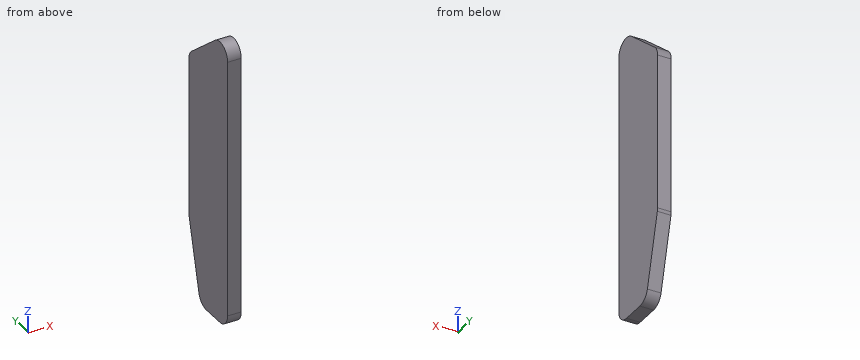
Autodesk Inventor part; units mm, degrees
ref_plane "YZ Plane" through (0, 0, 0) normal (1, 0, 0) x (0, 1, 0)
ref_plane "XZ Plane" through (0, 0, 0) normal (0, 1, 0) x (-1, 0, 0)
ref_plane "XY Plane" through (0, 0, 0) normal (0, 0, 1) x (1, 0, 0)
sketch "Sketch1" plane through (0, 0, 0) normal (1, 0, 0) x (0, 1, 0)
  line L0 (-15.875, 69.85) -> (15.875, 69.85)
  line L1 (15.875, 69.85) -> (15.875, -69.85)
  line L2 (15.875, -69.85) -> (-15.875, -69.85)
  line L3 (-15.875, -69.85) -> (-15.875, 69.85)
  line L4 (-15.875, 69.85) -> (15.875, -69.85) construction
  line L5 (15.875, 69.85) -> (-15.875, -69.85) construction
  line L6 (-15.875, 69.85) -> (15.875, 44.45)
  point P0 (0, 0)
  dimension "d0" = 31.75
  dimension "d1" = 139.7
  dimension "d2" = 25.4
extrude "Extrusion1" add sketch "Sketch1" along normal blind 6.35 contours L6 L1 L2 L3
chamfer "Chamfer1" distance 9.525 distance2 38.1 1 edges at (3.175, 15.875, -69.85) measured on face at (4.2333, -5.2917, -69.85)
fillet "Fillet1" radius 6.35 4 edges at (3.175, -15.875, 69.85) (3.175, 15.875, -31.75) (3.175, 6.35, -69.85) (3.175, -15.875, -69.85)
fillet "Fillet2" radius 6.35 1 edges at (3.175, 15.875, 44.45)
properties part number "Wheel Guards" material "UHMW, White"
Check sheet for the modelled part. Datum: model origin and axes. Units: mm. Coordinates: 2 decimals unless noted, no trailing zeros. Write each loop counter-clockwise with the first axis right and the second up, starting at its lowest first coordinate (ties: lowest second). Pieces come first, ordered by that corner, then holes. Notation, with made-up numbers: (-2, -25) - (5, -25) arc R25 cw to (5, -8) - close; hole circle Ø11 at (49.25, -12.75). An arc over 180 degrees is marked (long way). One line per question, with ' | ' between items.
Item 1: Gauge pin test, flat end, axial feed: P1, Ø1.5, axis at x = 3.5, z = -44.5, coming from the +Y side (3 decimals). Record the tip position at first contact, or that the pin passes through.
Determined:
P1: stops at y = 12.875
Item 2: Sectioned sample at A-A on x = 2. Record the boundary of the cut face in (y, z) (3 decimals), plus the area to 3 significant figures.
Determined:
outline: (-15.875, -63.5) arc R6.35 ccw to (-9.525, -69.85) - (1.392, -69.85) arc R6.35 ccw to (7.552, -65.04) - (15.685, -32.508) arc R6.35 ccw to (15.875, -30.968) - (15.875, 41.398) arc R6.35 ccw to (13.492, 46.357) - (-5.558, 61.597) arc R6.35 ccw to (-15.875, 56.638) - close | area: 3,800 mm2
Item 3: Thickness scan on line 1 (Z direction, x = 1.25, y = -10); line 2 (Y direction, x = 0.75, z = 47.5) (1 decimal); line 3 (Z direction, x = 3.5, y = 0.5). Record the ranges inside material, lowest first. Write a range as [from, to].
Determined:
line 1: z = [-69.83, 62.97] | line 2: y = [-15.9, 12.1] | line 3: z = [-69.85, 56.75]
Item 4: Sectioned sample at B-B on y = 11. Record the boundary of the cut face in (x, z).
Determined:
outline: (0, -51.25) - (6.35, -51.25) - (6.35, 48.35) - (0, 48.35) - close
